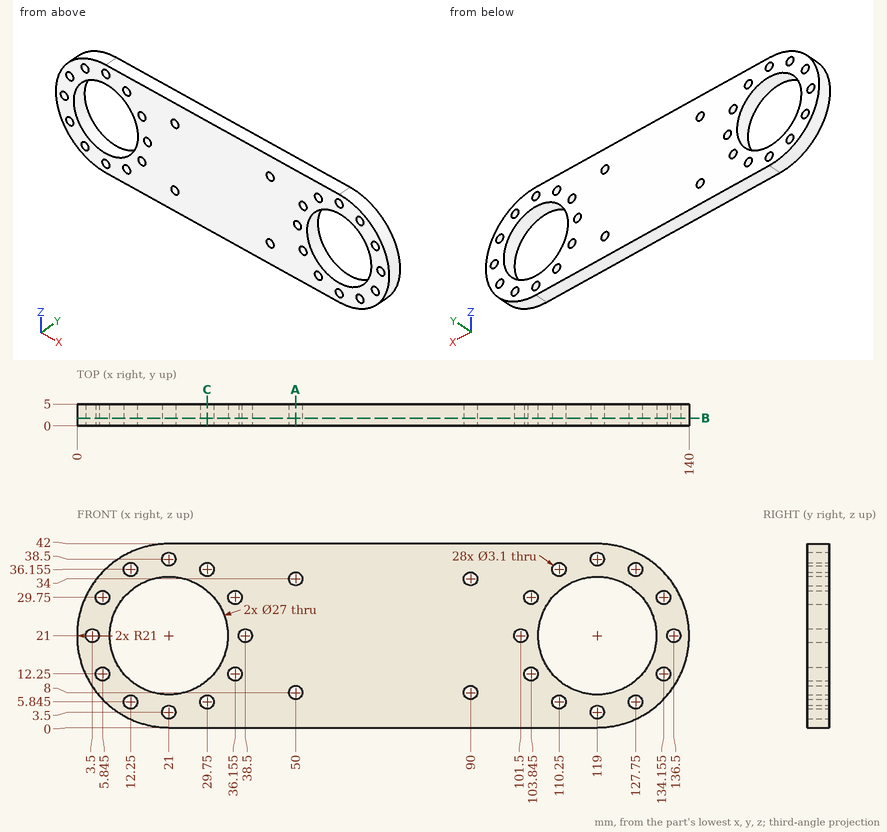
Study the drawing (mm; zero at the part's minimum x, y, z) and answer. Give positions to 0.01 mm unless a question says otherwise; leave off trailing zeros. Loops run counter-clockwise (first coordinate to the right, second up) from the corner with the lowest first, then second, coordinate; pieces in that order, holes last. Notation, with made-up numbers: (42, 64.5) -> (54, 64.5) arc R21 ccw to (54, 95.5) -> close; hole circle Ø7 at (31.25, 79). An arc over 180 degrees is marked (long way). Write item = value, one per line. Start each with the question number.
(1) Find the intervals of material crossed by probe 1 along Z at (x, y) = (119, 1.5); probe 2 along Z at (x, y) = (110.25, 3.75) (1 decimal); probe 3 along X at (y, z) = (2.3, 14) (1 decimal), in increasing order. Write a range as from..to.
(2) Find section A-A on x = 50. Give the vertices of the cut face in (y, z), and give its area (3 significant figures).
(3) Find section B-B on y = 1.75. Give the number of separate pieces and of enclosed holes in the cut face.
(4) Find section C-C on x = 29.75. Give the vertices of the cut face in (y, z) (1 decimal).
From the geometry:
q1.probe_1 = 0..1.95, 5.05..7.5, 34.5..36.95, 40.05..42
q1.probe_2 = 0..4.3, 7.4..10.7, 31.3..34.6, 37.7..42
q1.probe_3 = 1.2..9.5, 32.5..107.5, 130.5..138.8
q2.outline = (0, 0) -> (5, 0) -> (5, 6.45) -> (0, 6.45) -> close; (0, 9.55) -> (5, 9.55) -> (5, 32.45) -> (0, 32.45) -> close; (0, 35.55) -> (5, 35.55) -> (5, 42) -> (0, 42) -> close
q2.area = 179 mm^2
q3.separate_pieces = 1
q3.enclosed_holes = 30
q4.outline = (0, 0) -> (5, 0) -> (5, 4.3) -> (0, 4.3) -> close; (0, 7.4) -> (5, 7.4) -> (5, 10.7) -> (0, 10.7) -> close; (0, 31.3) -> (5, 31.3) -> (5, 34.6) -> (0, 34.6) -> close; (0, 37.7) -> (5, 37.7) -> (5, 42) -> (0, 42) -> close
